CAD build for the part. Positions are in the model's coordinates, mm. Give positions to 0.01 mm unless a question says otherwise; leave off trailing zeros. Write each loop counter-clockwise with the first axis right and the second up, starting at its lowest first coordinate (ties: lowest second). Pieces come first, ordered by that corner, then holes. Notation, with made-up numbers: (2.5, -16) -> (61.5, -16) arc R23 ccw to (61.5, 20) -> close; hole circle Ø11 at (35, 63). An arc over 180 degrees is marked (long way). Use one line per item in the form item = value. Start each with the question number.
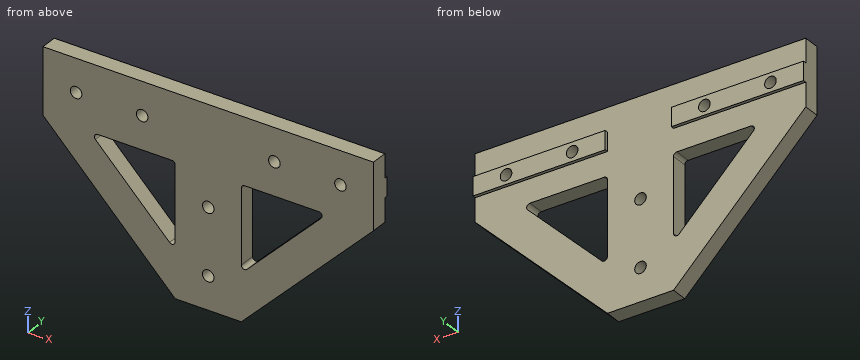
from build123d import *

# Parameters (mm, degrees)
ESBO_O1_R                = 1.75
RESSALTO_EXTRUS_O1_DEPTH = 5
ESBO_O3_W                = 40
ESBO_O3_H                = 5.65
ESBO_O3_R                = 1.75
RESSALTO_EXTRUS_O2_DEPTH = 1


with BuildPart() as part:
    # Esboço1 → Ressalto-extrusão1 (new body)
    with BuildSketch(Plane(origin=(0, 0, 0), x_dir=(1, 0, 0), z_dir=(0, 1, 0))):
        Polygon((-50, 0), (-50, 20.000002677), (-9.999996661, 60.000002546), (9.999996661, 60.000002546), (50, 20.000002677), (50, 0), align=None)
        with Locations(Location((-40, 10.000001339, 0), (0, 0, 270))):
            Circle(ESBO_O1_R, mode=Mode.SUBTRACT)
        with Locations(Location((-20, 10.000001339, 0), (0, 0, 270))):
            Circle(ESBO_O1_R, mode=Mode.SUBTRACT)
        with Locations(Location((0, 50.000002546, 0), (0, 0, 270))):
            Circle(ESBO_O1_R, mode=Mode.SUBTRACT)
        with Locations(Location((0, 30.000002546, 0), (0, 0, 270))):
            Circle(ESBO_O1_R, mode=Mode.SUBTRACT)
        with Locations(Location((20, 10.000001339, 0), (0, 0, 90))):
            Circle(ESBO_O1_R, mode=Mode.SUBTRACT)
        with Locations(Location((40, 10.000001339, 0), (0, 0, 90))):
            Circle(ESBO_O1_R, mode=Mode.SUBTRACT)
        with BuildLine():
            Line((-10, 43.443650782), (-10, 21.000001339))
            ThreePointArc((-10, 21.000001339), (-10.292893219, 20.292894558), (-11, 20.000001339))
            Line((-11, 20.000001339), (-33.443651391, 20.000001339))
            ThreePointArc((-33.443651391, 20.000001339), (-34.367530932, 20.617317926), (-34.150758141, 21.707108151))
            Line((-34.150758141, 21.707108151), (-11.707106751, 44.150757594))
            ThreePointArc((-11.707106751, 44.150757594), (-10.617316548, 44.367530307), (-10, 43.443650782))
        make_face(mode=Mode.SUBTRACT)
        with BuildLine():
            Line((11.707106751, 44.150757594), (34.150758141, 21.707108151))
            ThreePointArc((34.150758141, 21.707108151), (34.367530932, 20.617317926), (33.443651391, 20.000001339))
            Line((33.443651391, 20.000001339), (11, 20.000001339))
            ThreePointArc((11, 20.000001339), (10.292893219, 20.292894558), (10, 21.000001339))
            Line((10, 21.000001339), (10, 43.443650782))
            ThreePointArc((10, 43.443650782), (10.617316548, 44.367530307), (11.707106751, 44.150757594))
        make_face(mode=Mode.SUBTRACT)
    extrude(amount=RESSALTO_EXTRUS_O1_DEPTH)

    # Esboço3 → Ressalto-extrusão2 (add)
    # profile 1 of 2: a face of its own
    with BuildSketch(Plane(origin=(0, 5, 0), x_dir=(1, 0, 0), z_dir=(0, 1, 0))):
        with Locations((-30, 10.000001339)):
            Rectangle(ESBO_O3_W, ESBO_O3_H)
        with Locations(Location((-40, 10.000001339, 0), (0, 0, 270))):
            Circle(ESBO_O3_R, mode=Mode.SUBTRACT)
        with Locations(Location((-20, 10.000001339, 0), (0, 0, 270))):
            Circle(ESBO_O3_R, mode=Mode.SUBTRACT)
    # profile 2 of 2: a face of its own
    with BuildSketch(Plane(origin=(0, 5, 0), x_dir=(1, 0, 0), z_dir=(0, 1, 0))):
        with Locations((30, 10.000001339)):
            Rectangle(ESBO_O3_W, ESBO_O3_H)
        with Locations(Location((20, 10.000001339, 0), (0, 0, 90))):
            Circle(ESBO_O3_R, mode=Mode.SUBTRACT)
        with Locations(Location((40, 10.000001339, 0), (0, 0, 90))):
            Circle(ESBO_O3_R, mode=Mode.SUBTRACT)
    extrude(amount=RESSALTO_EXTRUS_O2_DEPTH)


solid = part.part
1) Cut at A-A (x = 40). Give the cut face in (y, z) (3 decimals), and give its area (3 significant figures).
2) Wall check: line 1 along X through (y, z) = (4.15, -10); line 2 along X through (y, z) = (1.25, -44); line 3 along Z through (x, y) = (20, 3.85). Give the ranges that are in metal, low to high. Write a range as from..to.
3) Pin check, flat tips, straight feed: pin 1 (18 mm diameter, centred on x = -0.5, z = -31, fed in from +Y); pin 2 (1 mm diameter, centred on y = 2, z = -31.5, fed in from -X); pin 3 (0.8 mm diameter, centred on x = 23.5, y = 5.5, fed in from -Z) (3 decimals). Stop position of each tip, or through.
4) Cut at D-D (z = -41). Give the cut face in (x, y).
5) Cut at C-C (x = 0). Give the cut face in (y, z), and give its area (3 significant figures).
6) Cut at B-B (y = 2). State how many separate pieces and enclosed holes the cut face has, and give its area (3 significant figures).
Final values:
q1.outline = (0, -30) -> (5, -30) -> (5, -12.825) -> (6, -12.825) -> (6, -11.75) -> (0, -11.75) -> close; (0, -8.25) -> (6, -8.25) -> (6, -7.175) -> (5, -7.175) -> (5, 0) -> (0, 0) -> close
q1.area = 135 mm^2
q2.line_1 = -50..-41.75, -38.25..-21.75, -18.25..18.25, 21.75..38.25, 41.75..50
q2.line_2 = -26..-11.86, -10.17..10.17, 11.86..26
q2.line_3 = -50..-35.86, -20..-11.75, -8.25..0
q3.pin_1 = 5
q3.pin_2 = -39
q3.pin_3 = -12.825
q4.outline = (-29, 0) -> (-14.86, 0) -> (-14.86, 5) -> (-29, 5) -> close; (-10, 0) -> (10, 0) -> (10, 5) -> (-10, 5) -> close; (14.86, 0) -> (29, 0) -> (29, 5) -> (14.86, 5) -> close
q5.outline = (0, -60) -> (5, -60) -> (5, -51.75) -> (0, -51.75) -> close; (0, -48.25) -> (5, -48.25) -> (5, -31.75) -> (0, -31.75) -> close; (0, -28.25) -> (5, -28.25) -> (5, 0) -> (0, 0) -> close
q5.area = 265 mm^2
q6.separate_pieces = 1
q6.enclosed_holes = 8
q6.area = 3,680 mm^2
